```python
from build123d import *

# Parameters (mm, degrees)
F0_W     = 50
F0_H     = 50
F1_DEPTH = 225
F2_R     = 4
F3_DEPTH = 25
F4_R     = 4
F5_DEPTH = 25


with BuildPart() as f1:
    # F0 (on Right) → F1 (new body, symmetric)
    with BuildSketch(Plane.YZ):
        Rectangle(F0_W, F0_H)
    extrude(amount=F1_DEPTH, both=True)

    # F2 (on face) → F3 (cut)
    with BuildSketch(Plane.YZ.offset(225)):
        with Locations((-10, 10)):
            Circle(F2_R)
        with Locations((10, 10)):
            Circle(F2_R)
        with Locations((10, -10)):
            Circle(F2_R)
        with Locations((-10, -10)):
            Circle(F2_R)
    extrude(amount=-F3_DEPTH, mode=Mode.SUBTRACT)

    # F4 (on face) → F5 (cut)
    with BuildSketch(Plane(origin=(-225, 0, 0), x_dir=(0, -1, 0), z_dir=(-1, 0, 0))):
        with Locations((-10, 10)):
            Circle(F4_R)
        with Locations((10, 10)):
            Circle(F4_R)
        with Locations((10, -10)):
            Circle(F4_R)
        with Locations((-10, -10)):
            Circle(F4_R)
    extrude(amount=-F5_DEPTH, mode=Mode.SUBTRACT)


solid = f1.part
```
Work out the finished part from the listing and answer in its coordinate system (mm). A direction names the side the tool comes from. Round coordinates to 2 decimals unless told otherwise and drop trailing zeros. Write each loop counter-clockwise with the first axis right and the second up, starting at its lowest first coordinate (ties: lowest second). Pieces come first, ordered by that corner, then holes. Notation, with made-up numbers: (50, 78) -> (73, 78) arc R32 cw to (73, 109) -> close; hole circle Ø10 at (41.25, 64.25). An arc over 180 degrees is marked (long way). Write each question's results on one line, items separated by ' | '.
1) The part is cut by section A-A (z = 10). Write down the section's boundary in (x, y), and give its area (3 significant figures).
Findings:
outline: (-225, -25) -> (225, -25) -> (225, -14) -> (200, -14) -> (200, -6) -> (225, -6) -> (225, 6) -> (200, 6) -> (200, 14) -> (225, 14) -> (225, 25) -> (-225, 25) -> (-225, 14) -> (-200, 14) -> (-200, 6) -> (-225, 6) -> (-225, -6) -> (-200, -6) -> (-200, -14) -> (-225, -14) -> close | area: 21,700 mm²
2) Which of the six approach directions +Z, -Z, +X, -X, +Y, -Y give full straight-line access (tool end or side, diameter ignored) to faces 1 (the flat face through (3, 0, 25)), 2 (the flat face through (200, 10, 10)), 3 (the flat face through (-200, -10, 10))?
Findings:
face 1: +Z, +X, -X, +Y, -Y | face 2: +X | face 3: -X
3) Consider line 1 along Z through (x, y) = (212, -10); line 2 along Y through (x, z) = (-205, -12.5); line 3 along X through (y, z) = (-9, 9). Determine where each line is inside the solid, lowest interval first. Write a range as [from, to].
Findings:
line 1: z = [-25, -14], [-6, 6], [14, 25] | line 2: y = [-25, -13.12], [-6.88, 6.88], [13.12, 25] | line 3: x = [-200, 200]
4) Flat-ended cylindrical pins translate along their axes: pin 1 (3 mm diameter, centred on y = 9, z = 11, fed in from -X); pin 2 (4 mm diameter, centred on y = 9, z = 10.5, fed in from +X). Find the tip coordinate at first contact, or state that the pin passes through.
Findings:
pin 1: stops at x = -200 | pin 2: stops at x = 200
5) For a pull along Y with two mould halves and no side action, classify faces 4 (the cylindrical face through (-213, -6, 10)), 5 (the flat face through (225, 0, 0)), 6 (the flat face through (3, -25, 0)) as +Y half, -Y half, draft (parallel to the pull), parting line (faces both ways), or undercut.
Findings:
face 4: undercut | face 5: draft | face 6: -Y half
